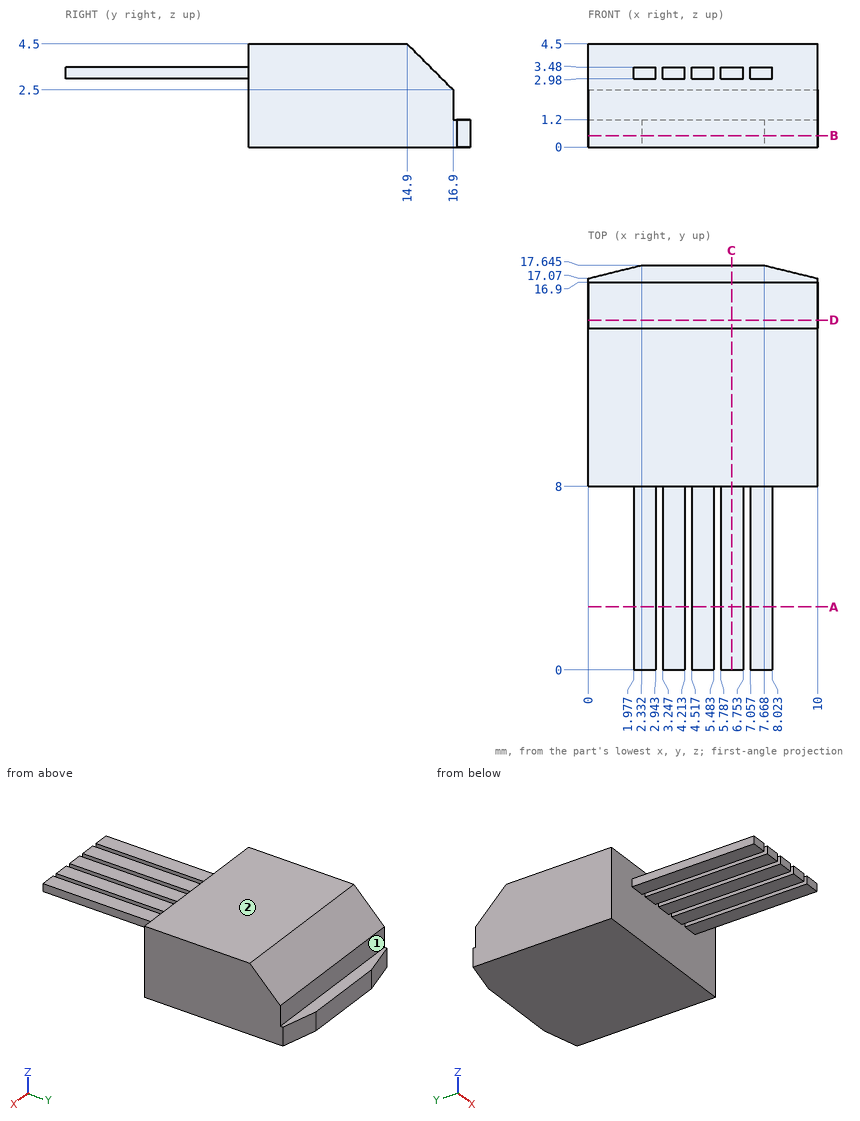
Check sheet for the drawn part. Datum: minimum x, y, z corner. Units: mm. A direction names the side the tool comes from. Round coordinates to 2 decimals unless told otherwise and drop trailing zeros. Loops run counter-clockwise (first coordinate to the right, second up) from the corner with the lowest first, then second, coordinate; pieces in that order, holes last. Notation, with made-up numbers: (-1, 70) -> (58, 70) arc R22 cw to (58, 103) -> close; hole circle Ø9 at (40, -8). An arc over 180 degrees is marked (long way). Put each result on its own line as item: value. Start each with the question number.
1. Gauge pin test, flat ends, axial feed: pin 1 (1.1 mm diameter, centred on x = 2.5, y = 4.5, fed in from -Z); pin 2 (0.8 mm diameter, centred on x = 6, y = 5, fed in from +Z); pin 3 (1.3 mm diameter, centred on x = 3.5, z = 1.5, fed in from -Y); pin 4 (3 mm diameter, centred on x = 3, y = 9, fed in from -Z). Record the tip position at first contact, or that the pin passes through.
2. Section check D-D (y = 15.25). Enter the section's corners in (x, z).
3. Section check B-B (z = 0.5). Enter the section's corners in (x, y) (1 decimal).
4. Scan lines: probe 1 along Z at (x, y) = (7.5, 6.5); probe 2 along Y at (x, z) = (3.25, 1.9); probe 3 along Z at (x, y) = (7.75, 16). Record each from-to range of solid material in increasing order.
5. Section check C-C (x = 6.25). Enter the section's corners in (y, z) (1 decimal).
6. Section check A-A (y = 2.75). Enter the section's corners in (x, z).
7. Access from +Z, -Z, +X, -X, +Y, -Y to the whole of each face (thin tool, end or side, straight path). Record for the marked faces 1 and 2.
Findings:
1. pin 1: stops at z = 2.98
1. pin 2: stops at z = 3.48
1. pin 3: stops at y = 8
1. pin 4: stops at z = 0
2. outline: (0, 0) -> (10, 0) -> (10, 4.15) -> (0, 4.15) -> close
3. outline: (0, 8) -> (10, 8) -> (10, 17.1) -> (7.7, 17.6) -> (2.3, 17.6) -> (0, 17.1) -> close
4. probe 1: z = 2.98 to 3.48
4. probe 2: y = 8 to 16.9
4. probe 3: z = 0 to 3.4
5. outline: (0, 3) -> (8, 3) -> (8, 0) -> (17.6, 0) -> (17.6, 1.2) -> (16.9, 1.2) -> (16.9, 2.5) -> (14.9, 4.5) -> (8, 4.5) -> (8, 3.5) -> (0, 3.5) -> close
6. outline: (1.98, 2.98) -> (2.94, 2.98) -> (2.94, 3.48) -> (1.98, 3.48) -> close; (3.25, 2.98) -> (4.21, 2.98) -> (4.21, 3.48) -> (3.25, 3.48) -> close; (4.52, 2.98) -> (5.48, 2.98) -> (5.48, 3.48) -> (4.52, 3.48) -> close; (5.79, 2.98) -> (6.75, 2.98) -> (6.75, 3.48) -> (5.79, 3.48) -> close; (7.06, 2.98) -> (8.02, 2.98) -> (8.02, 3.48) -> (7.06, 3.48) -> close
7. face 1: +Z, +X, -X, +Y
7. face 2: +Z, +X, -X, +Y, -Y
